Read the model definition and answer for the solid it produces. Units are mm, in the model's axes. Coordinates: 2 decimals unless noted, no trailing zeros. Loops run counter-clockwise (first coordinate to the right, second up) from the corner with the lowest first, then second, coordinate; pieces in that order, holes last. Notation, with made-up numbers: (45, 48) - (55, 48) arc R36 cw to (55, 87) - close; hole circle Ø11 at (-32, 39.25). An arc over 180 degrees is marked (long way). One line per question, with ' | ' between items. Start each with the question number.
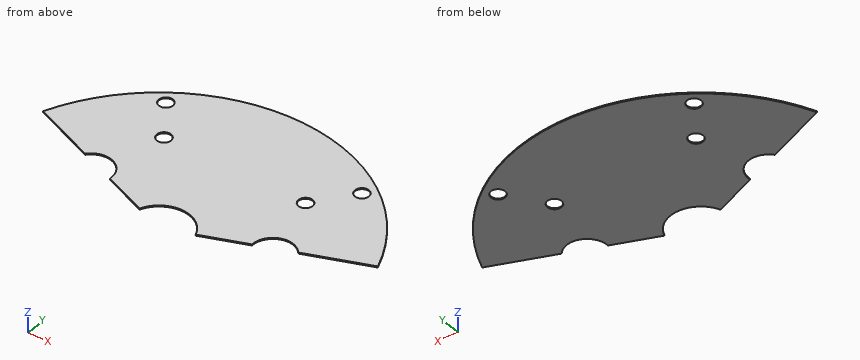
```python
from build123d import *

# Parameters (mm, degrees)
BOSS_EXTRUDE1_DEPTH = 0.3
SKETCH7_R           = 1.905
CUT_EXTRUDE2_DEPTH  = 68.300419328
CUT_EXTRUDE3_DEPTH  = 68.300419328


with BuildPart() as part:
    # Sketch5 → Boss-Extrude1 (new body)
    with BuildSketch(Plane.XY):
        with BuildLine():
            Line((-7.679064705, 3.029354759), (-45.838109317, 18.082917637))
            ThreePointArc((-45.838109317, 18.082917637), (-28.963706092, 39.865121415), (-3.033121883, 49.182561418))
            ThreePointArc((-3.033121883, 49.182561418), (26.454937122, 41.572352326), (45.838109317, 18.082917637))
            Line((45.838109317, 18.082917637), (7.679064705, 3.029354759))
            ThreePointArc((7.679064705, 3.029354759), (4.431883796, 6.964440467), (-0.508126089, 8.239346629))
            ThreePointArc((-0.508126089, 8.239346629), (-4.852167258, 6.678435289), (-7.679064705, 3.029354759))
        make_face()
    extrude(amount=BOSS_EXTRUDE1_DEPTH)

    # Sketch7 → Cut-Extrude2 (cut, through all)
    with BuildSketch(Plane(origin=(0, 0, 0), x_dir=(-1, 0, 0), z_dir=(0, 0, -1))):
        with Locations((-26.813856327, 36.919157691)):
            Circle(SKETCH7_R)
        with Locations((-19.358590444, 26.657864517)):
            Circle(SKETCH7_R)
        with Locations((26.838840816, 36.900999332)):
            Circle(SKETCH7_R)
        with Locations((19.383574933, 26.639706158)):
            Circle(SKETCH7_R)
    extrude(amount=-CUT_EXTRUDE2_DEPTH, mode=Mode.SUBTRACT)

    # Sketch8 → Cut-Extrude3 (cut, through all)
    with BuildSketch(Plane(origin=(0, 0, 0), x_dir=(-1, 0, 0), z_dir=(0, 0, -1))):
        with BuildLine():
            Line((-19.468246955, 7.680131477), (-29.179148849, 11.511036411))
            ThreePointArc((-29.179148849, 11.511036411), (-22.930885785, 13.12620192), (-19.468246955, 7.680131477))
        make_face()
        with BuildLine():
            Line((29.183436436, 11.512727844), (19.425492338, 7.663264983))
            ThreePointArc((19.425492338, 7.663264983), (22.882252084, 13.193140466), (29.183436436, 11.512727844))
        make_face()
    extrude(amount=-CUT_EXTRUDE3_DEPTH, mode=Mode.SUBTRACT)


solid = part.part
```
1) The part is cut by section B-B on z = 0.15. Write down the section's boundary in (x, y) (1 decimal).
2) The part is cut by section D-D on x = -38. Write down the section's boundary in (y, z), and give its area (3 significant figures).
3) Given pin 1 Ø6 at (x, y) = (19.36, 26.66) entering from -Z, flat-ended and moving along its own axis, determine where the tip first touches the part or whether it passes through.
4) The part is cut by section C-C on y = 16.5. Write down the section's boundary in (x, z), and give its area (3 significant figures).
5) The part is cut by section A-A on x = -18.5. Write down the section's boundary in (y, z).
6) Find the intervals of material crossed by line 1 along Y through (x, z) = (18, 0.2); line 2 along Y through (x, z) = (3, 0.2); line 3 along Y through (x, z) = (-14.5, 0.2), in increasing order. Write a range as from..to.
Answer below:
1) outline: (-45.8, 18.1) - (-29.2, 11.5) arc R5.5 cw to (-19.4, 7.7) - (-7.7, 3) arc R8.3 cw to (7.7, 3) - (19.5, 7.7) arc R5.5 cw to (29.2, 11.5) - (45.8, 18.1) arc R49.3 ccw to start; hole circle Ø3.8 at (-26.8, 36.9); hole circle Ø3.8 at (-19.4, 26.6); hole circle Ø3.8 at (19.4, 26.7); hole circle Ø3.8 at (26.8, 36.9)
2) outline: (14.99, 0) - (31.37, 0) - (31.37, 0.3) - (14.99, 0.3) - close | area: 4.91 mm2
3) pin 1: z = 0
4) outline: (-41.83, 0) - (41.83, 0) - (41.83, 0.3) - (-41.83, 0.3) - close | area: 25.1 mm2
5) outline: (7.3, 0) - (24.95, 0) - (24.95, 0.3) - (7.3, 0.3) - close; (28.33, 0) - (45.67, 0) - (45.67, 0.3) - (28.33, 0.3) - close
6) line 1: 7.1..25.32, 27.99..45.87 | line 2: 7.69..49.18 | line 3: 5.72..47.09
